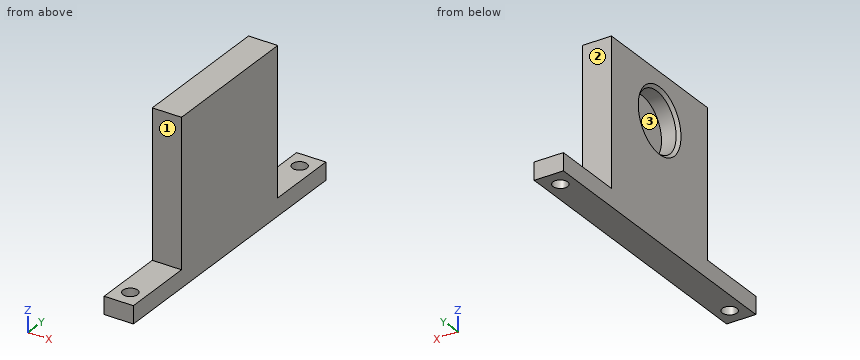
```python
from build123d import *

# Parameters (mm, degrees)
EXTRUDE_2_DEPTH     = 5
SKETCH_2_R          = 1.25
CUT_EXTRUDE_1_DEPTH = 4
SKETCH_3_R          = 5.05
CUT_EXTRUDE_2_DEPTH = 3
CHAMFER_1_SIZE      = 0.5


with BuildPart() as part:
    # 草图1 → 凸台-拉伸2 (new body)
    with BuildSketch(Plane(origin=(0, 0, 0), x_dir=(0, 0, -1), z_dir=(1, 0, 0))):
        Polygon((25, 25), (25, 37.5), (28, 37.5), (28, -12.5), (25, -12.5), (25, 0), (0, 0), (0, 25), align=None)
    extrude(amount=EXTRUDE_2_DEPTH)

    # 草图2 → 切除-拉伸1 (cut)
    with BuildSketch(Plane.XY.offset(-25)):
        with Locations((2.5, 34.5)):
            Circle(SKETCH_2_R)
        with Locations((2.5, -9.5)):
            Circle(SKETCH_2_R)
    extrude(amount=-CUT_EXTRUDE_1_DEPTH, mode=Mode.SUBTRACT)

    # 草图3 → 切除-拉伸2 (cut)
    with BuildSketch(Plane.ZY):
        with Locations((-8, 12.5)):
            Circle(SKETCH_3_R)
    extrude(amount=-CUT_EXTRUDE_2_DEPTH, mode=Mode.SUBTRACT)

    # 倒角1
    chamfer_1_edges = [part.edges().sort_by_distance(p)[0] for p in [
        (0, 12.5, -13.05),
    ]]
    chamfer(chamfer_1_edges, length=CHAMFER_1_SIZE)


solid = part.part
```
Check sheet for the modelled part. Datum: model origin and axes. Units: mm. Face numbers are marked on the shaded views. A direction names the side the tool comes from. Give positions to 0.01 mm unless a question says otherwise; leave off trailing zeros. Order: outer loops, then holes, each group sorted by start corner. A loop starts at its lowest first (then second) coordinate and runs counter-clockwise, first axis right, second up. Notation, with made-up numbers: (61, 25) -> (115, 25) arc R9 ccw to (115, 34) -> close; hole circle Ø5 at (78, 25.5). An arc over 180 degrees is marked (long way). Use CSV: the item, a comma, the result in double quotes. Start each with the question number.
1) Sectioned sample at B-B, the plane y = 34.5. Record the boundary of the cut face in (x, z), plus the area to 3 significant figures.
2) Sectioned sample at C-C, the plane z = -8. Record the boundary of the cut face in (x, y), plus the area to 4 significant figures.
3) Sectioned sample at D-D, the plane y = 12.5. Record the boundary of the cut face in (x, z).
4) Material ranges on line 1 (Y direction, x = 2.5, z = -26.85); line 2 (Y direction, x = 1.15, z = -8); line 3 (Y direction, x = 2.9, z = -23.25), recorded low to high. Write a range as from..to.
5) Set-up check for the marked faces 1, 2 and 3: record each of +Z, -Z, +X, -X, +Y, -Y from which the full face is reachable in a straight line by a thin tool's end or side.
6) Sectioned sample at A-A, the plane x = 2.5. Record the boundary of the cut face in (y, z), plus the area to 3 significant figures.
7) Go/stop test with flat-tipped pins: P1, Ø1.5, axis at x = 1.5, z = -13.5, coming from the -Y side; P2, Ø3, axis at x = 2.5, y = 34.5, coming from the +Z side; P3, Ø3, axis at x = 2, z = -13, coming from the +Y side. Record where each tip stops, or that it passes through.
Recorded:
1,outline,"(0, -28) -> (1.25, -28) -> (1.25, -25) -> (0, -25) -> close; (3.75, -28) -> (5, -28) -> (5, -25) -> (3.75, -25) -> close"
1,area,"7.50 mm2"
2,outline,"(0, 0) -> (5, 0) -> (5, 25) -> (0, 25) -> (0, 18.05) -> (0.5, 17.55) -> (3, 17.55) -> (3, 7.45) -> (0.5, 7.45) -> (0, 6.95) -> close"
2,area,"94.45 mm2"
3,outline,"(0, -28) -> (5, -28) -> (5, 0) -> (0, 0) -> (0, -2.45) -> (0.5, -2.95) -> (3, -2.95) -> (3, -13.05) -> (0.5, -13.05) -> (0, -13.55) -> close"
4,line 1,"-12.5..-10.75, -8.25..33.25, 35.75..37.5"
4,line 2,"0..7.45, 17.55..25"
4,line 3,"0..25"
5,face 1,"+Z, +X, -X, -Y"
5,face 2,"+Z, +X, -X, +Y"
5,face 3,"-X"
6,outline,"(-12.5, -28) -> (-10.75, -28) -> (-10.75, -25) -> (-12.5, -25) -> close; (-8.25, -28) -> (33.25, -28) -> (33.25, -25) -> (25, -25) -> (25, 0) -> (0, 0) -> (0, -25) -> (-8.25, -25) -> close; (35.75, -28) -> (37.5, -28) -> (37.5, -25) -> (35.75, -25) -> close; hole circle Ø10.1 at (12.5, -8)"
6,area,"680 mm2"
7,P1,"y = 0"
7,P2,"z = -25"
7,P3,"y = 25"
